from build123d import *

# Parameters (mm, degrees)
BOSS_EXTRUDE1_DEPTH = 2.54
SKETCH2_W           = 5.08
SKETCH2_H           = 20.32
BOSS_EXTRUDE2_DEPTH = 2.54
SKETCH3_R           = 1.524
CUT_EXTRUDE1_DEPTH  = 2.54


with BuildPart() as part:
    # Sketch1 → Boss-Extrude1 (new body)
    with BuildSketch(Plane.XY):
        Polygon((-8.89, 0), (-8.89, 7.62), (8.89, 7.62), (8.89, 5.08), (12.681599437, 0), (16.473198875, 5.08), (20.264798312, 0), (24.056397749, 5.08), (27.847997187, 0), (31.639596624, 5.08), (35.431196061, 0), (39.222795499, 5.08), (43.014394936, 0), (46.99, 5.08), (46.99, 0), (46.99, -2.620396656), (-8.89, -2.620396656), align=None)
    extrude(amount=BOSS_EXTRUDE1_DEPTH)

    # Sketch2 → Boss-Extrude2 (add)
    with BuildSketch(Plane.ZY.offset(8.89)):
        with Locations((1.27, 2.459603344)):
            Rectangle(SKETCH2_W, SKETCH2_H)
    extrude(amount=BOSS_EXTRUDE2_DEPTH)

    # Sketch3 → Cut-Extrude1 (cut)
    with BuildSketch(Plane.ZY.offset(11.43)):
        with Locations((1.27, 10.333603344)):
            Circle(SKETCH3_R)
        with Locations(Location((1.27, -5.414396656, 0), (0, 0, 180))):
            Circle(SKETCH3_R)
    extrude(amount=-CUT_EXTRUDE1_DEPTH, mode=Mode.SUBTRACT)


solid = part.part
Source: CAD feature listing. Evaluate the final solid. Frame: model axes, mm. A direction names the side the tool comes from. Give positions to 0.01 mm unless a question says otherwise; leave off trailing zeros. Write each loop counter-clockwise with the first axis right and the second up, starting at its lowest first coordinate (ties: lowest second). Pieces come first, ordered by that corner, then holes. Notation, with made-up numbers: M 56,37.25 L 60,37.25 A26 cw 60,58.25 Z; hole C -39,81 d3. An arc over 180 degrees is marked long. Return JSON: item names as keys, results as strings. Group by question number.
1) Draft query along Y for faces 5 (the face through (-10, -7.7, 1)), 6 (the face through (-10.178, 11.845, 1.072)), 7 (the face through (22.13, 2.5, 1.25)). Return one class per face: released by +Y, released by -Y, zero draft, split by the parting line, or undercut.
2) Cut plane D-D, the plane y = 0.75. Output: boundary loops of the cut face in (x, z).
3) Ray query, L1, parallel to Y at x = -10.3, z = 1.27; L2, parallel to X at y = 4.5, z = 1.9; L3, parallel to X at y = 9, z = -0.9. Return the intervals inside material, ascending.
4) Cut plane A-A, the plane z = 1.27. Output: boundary loops of the cut face in (x, y).
5) First-contact query: pin 1 Ø3 at (x, y) = (7.5, 2.5) entering from +Z; pin 2 Ø3 at (x, y) = (26.5, 0.5) entering from -Z; pin 3 Ø2 at (y, z) = (6.5, 0.5) entering from +X. Flat tips, straight axial feed; report the tip coordinate or a pass-through.
6) Set-up query: faces 1 (the face through (19, -2.62, 1)), 2 (the face through (29.717, 2.504, 1.252)), 3 (the face through (13, 0, 0)), 4 (the face through (13, 0, 2.54)). Return all of +Z, -Z, +X, -X, +Y, -Y with unobstructed straight access to the full face (end or side cutting, diameter ignored); none if empty.
7) Cut plane B-B, the plane y = 4. Output: boundary loops of the cut face in (x, z), then the cut area to 3 significant figures.
8) Cut plane C-C, the plane x = 1. Output: boundary loops of the cut face in (y, z), then the cut area to 3 significant figures.
Data:
{
 "1": {"face 5": "released by -Y", "face 6": "undercut", "face 7": "released by +Y"},
 "2": {"outline": "M -11.43,-1.27 L -8.89,-1.27 L -8.89,0 L 12.12,0 L 12.12,2.54 L -8.89,2.54 L -8.89,3.81 L -11.43,3.81 Z; M 13.24,0 L 19.71,0 L 19.71,2.54 L 13.24,2.54 Z; M 20.82,0 L 27.29,0 L 27.29,2.54 L 20.82,2.54 Z; M 28.41,0 L 34.87,0 L 34.87,2.54 L 28.41,2.54 Z; M 35.99,0 L 42.45,0 L 42.45,2.54 L 35.99,2.54 Z; M 43.6,0 L 46.99,0 L 46.99,2.54 L 43.6,2.54 Z"},
 "3": {"L1": "y = -7.7 to -6.94, -3.89 to 8.81, 11.86 to 12.62", "L2": "x = -11.43 to 9.32, 16.04 to 16.91, 23.62 to 24.49, 31.21 to 32.07, 38.79 to 39.66, 46.54 to 46.99", "L3": "x = -11.43 to -8.89"},
 "4": {"outline": "M -11.43,-7.7 L -8.89,-7.7 L -8.89,-6.94 L -11.43,-6.94 Z; M -11.43,-3.89 L -8.89,-3.89 L -8.89,-2.62 L 46.99,-2.62 L 46.99,5.08 L 43.01,0 L 39.22,5.08 L 35.43,0 L 31.64,5.08 L 27.85,0 L 24.06,5.08 L 20.26,0 L 16.47,5.08 L 12.68,0 L 8.89,5.08 L 8.89,7.62 L -8.89,7.62 L -8.89,8.81 L -11.43,8.81 Z; M -11.43,11.86 L -8.89,11.86 L -8.89,12.62 L -11.43,12.62 Z"},
 "5": {"pin 1": "stops at z = 2.54", "pin 2": "stops at z = 0", "pin 3": "stops at x = 8.89"},
 "6": {"face 1": "+Z, -Z, +X, -Y", "face 2": "+Z, -Z, +Y", "face 3": "-Z, +X, +Y, -Y", "face 4": "+Z, +X, +Y, -Y"},
 "7": {"outline": "M -11.43,-1.27 L -8.89,-1.27 L -8.89,0 L 9.7,0 L 9.7,2.54 L -8.89,2.54 L -8.89,3.81 L -11.43,3.81 Z; M 15.67,0 L 17.28,0 L 17.28,2.54 L 15.67,2.54 Z; M 23.25,0 L 24.86,0 L 24.86,2.54 L 23.25,2.54 Z; M 30.83,0 L 32.45,0 L 32.45,2.54 L 30.83,2.54 Z; M 38.42,0 L 40.03,0 L 40.03,2.54 L 38.42,2.54 Z; M 46.14,0 L 46.99,0 L 46.99,2.54 L 46.14,2.54 Z", "area": "78.6 mm²"},
 "8": {"outline": "M -2.62,0 L 7.62,0 L 7.62,2.54 L -2.62,2.54 Z", "area": "26.0 mm²"}
}
